from build123d import *

# Parameters (mm, degrees)
SKETCH1_W           = 5
SKETCH1_H           = 85
BOSS_EXTRUDE1_DEPTH = 95
SKETCH2_W           = 85
SKETCH2_H           = 5
BOSS_EXTRUDE2_DEPTH = 10
SKETCH3_W           = 30
SKETCH3_H           = 30
CUT_EXTRUDE1_DEPTH  = 10


with BuildPart() as part:
    # Sketch1 → Boss-Extrude1 (new body)
    with BuildSketch(Plane(origin=(0, 0, 0), x_dir=(1, 0, 0), z_dir=(0, 1, 0))):
        with Locations((-2.5, -42.5)):
            Rectangle(SKETCH1_W, SKETCH1_H)
    extrude(amount=BOSS_EXTRUDE1_DEPTH)

    # Sketch2 → Boss-Extrude2 (add)
    with BuildSketch(Plane.ZY.offset(5)):
        with Locations((42.5, 92.5)):
            Rectangle(SKETCH2_W, SKETCH2_H)
    extrude(amount=BOSS_EXTRUDE2_DEPTH)

    # Sketch3 → Cut-Extrude1 (cut)
    with BuildSketch(Plane.ZY.offset(5)):
        with Locations((42.573593129, 42.5)):
            Rectangle(SKETCH3_W, SKETCH3_H)
    extrude(amount=-CUT_EXTRUDE1_DEPTH, mode=Mode.SUBTRACT)


solid = part.part
Geometry: final body of the model. Coordinates: model frame, mm. A direction names the side the tool comes from. Coordinates: 2 decimals unless noted, no trailing zeros. Loops run counter-clockwise (first coordinate to the right, second up) from the corner with the lowest first, then second, coordinate; pieces in that order, holes last. Notation, with made-up numbers: (88.25, 18) - (135.25, 18) arc R34 ccw to (135.25, 57) - close; hole circle Ø6 at (-21, 5). An arc over 180 degrees is marked (long way). Put each result on its own line as item: value. Start each with the question number.
Q1. Cut plane A-A, the plane z = 38. Return loops of the section in (x, y), and give its area (3 significant figures).
Q2. Line query: line 1 (Y direction, x = -4.75, z = 48.5); line 2 (Z direction, x = -3.25, y = 38.5); line 3 (Y direction, x = -13.25, z = 72). Output: solid intervals per line, ascending.
Q3. Cut plane D-D, the plane x = -10. Return loops of the section in (y, z).
Q4. Cut plane C-C, the plane z = 17. Return loops of the section in (x, y).
Q5. Pull-direction query (Z, two-part tool) for faces 4 (the flat face through (-3, 27.5, 42)), 5 (the flat face through (-4, 51, 0)), 6 (the flat face through (-3, 0, 42)); classes: released by +Z, released by -Z, zero draft, split by the parting line, or undercut.
Q6. Set-up query: faces 1 (the flat face through (-3, 42, 57.574)), 2 (the flat face through (-10, 90, 42)), 3 (the flat face through (-15, 93, 42)). Return all of +Z, -Z, +X, -X, +Y, -Y with unobstructed straight access to the full face (end or side cutting, diameter ignored); none if empty.
Q7. Pin query (flat end, axial travel): pin 1 Ø2 at (y, z) = (61, 62) entering from +X; pin 2 Ø5 at (x, z) = (-10, 24.5) entering from -Y. Return the tip coordinate at first contact, or that it passes through.
Q8. Cut plane B-B, the plane x = -2. Return loops of the section in (y, z), and give its area (4 significant figures).
Filled sheet:
1. outline: (-15, 90) - (-5, 90) - (-5, 57.5) - (0, 57.5) - (0, 95) - (-15, 95) - close; (-5, 0) - (0, 0) - (0, 27.5) - (-5, 27.5) - close
1. area: 375 mm²
2. line 1: 0 to 27.5, 57.5 to 95
2. line 2: 0 to 27.57, 57.57 to 85
2. line 3: 90 to 95
3. outline: (90, 0) - (95, 0) - (95, 85) - (90, 85) - close
4. outline: (-15, 90) - (-5, 90) - (-5, 0) - (0, 0) - (0, 95) - (-15, 95) - close
5. face 4: undercut
5. face 5: released by -Z
5. face 6: zero draft
6. face 1: +X, -X
6. face 2: +Z, -Z, -X, -Y
6. face 3: +Z, -Z, -X, +Y, -Y
7. pin 1: x = 0
7. pin 2: y = 90
8. outline: (0, 0) - (95, 0) - (95, 85) - (0, 85) - close; hole (27.5, 27.57) - (57.5, 27.57) - (57.5, 57.57) - (27.5, 57.57) - close
8. area: 7,175 mm²
